from build123d import *

# Parameters (mm, degrees)
F0_W     = 42.2
F0_H     = 42
F1_DEPTH = 6
F3_R     = 1
F4_R     = 1
F5_DEPTH = 3
F6_R     = 1.65
F7_DEPTH = 6.001


with BuildPart() as f1:
    # F0 (on Top) → F1 (new body)
    with BuildSketch(Plane.XY):
        Rectangle(F0_W, F0_H)
        with BuildLine():
            Line((13, -8), (-13, -8))
            ThreePointArc((-13, -8), (-15.5, -5.5), (-13, -3))
            Line((-13, -3), (13, -3))
            ThreePointArc((13, -3), (15.5, -5.5), (13, -8))
        make_face(mode=Mode.SUBTRACT)
        with BuildLine():
            Line((13, 3), (-13, 3))
            ThreePointArc((-13, 3), (-15.5, 5.5), (-13, 8))
            Line((-13, 8), (13, 8))
            ThreePointArc((13, 8), (15.5, 5.5), (13, 3))
        make_face(mode=Mode.SUBTRACT)
    extrude(amount=F1_DEPTH)

    # F3
    f3_edges = [f1.edges().sort_by_distance(p)[0] for p in [
        (-21.1, -21, 3),
        (21.1, -21, 3),
        (-21.1, 21, 3),
        (21.1, 21, 3),
    ]]
    fillet(f3_edges, radius=F3_R)

    # F4
    f4_edges = [f1.edges().sort_by_distance(p)[0] for p in [
        (0, -21, 0),
        (0, -3, 0),
        (0, 8, 0),
    ]]
    fillet(f4_edges, radius=F4_R)

    # F2 (on face) → F5 (cut)
    with BuildSketch(Plane(origin=(0, 0, 0), x_dir=(1, 0, 0), z_dir=(0, 0, -1))):
        Polygon((-12.5, 13.767949), (-12.5, 17.232051), (-15.5, 18.964102), (-18.5, 17.232051), (-18.5, 13.767949), (-15.5, 12.035898), align=None)
        Polygon((12.5, 17.232051), (12.5, 13.767949), (15.5, 12.035898), (18.5, 13.767949), (18.5, 17.232051), (15.5, 18.964102), align=None)
        Polygon((12.5, -13.767949), (12.5, -17.232051), (15.5, -18.964102), (18.5, -17.232051), (18.5, -13.767949), (15.5, -12.035898), align=None)
        Polygon((-12.5, -17.232051), (-12.5, -13.767949), (-15.5, -12.035898), (-18.5, -13.767949), (-18.5, -17.232051), (-15.5, -18.964102), align=None)
    extrude(amount=-F5_DEPTH, mode=Mode.SUBTRACT)

    # F6 (on face) → F7 (cut, through all)
    with BuildSketch(Plane(origin=(0, 0, 0), x_dir=(1, 0, 0), z_dir=(0, 0, -1))):
        with Locations((-15.5, 15.5)):
            Circle(F6_R)
        with Locations((15.5, 15.5)):
            Circle(F6_R)
        with Locations((15.5, -15.5)):
            Circle(F6_R)
        with Locations((-15.5, -15.5)):
            Circle(F6_R)
    extrude(amount=-F7_DEPTH, mode=Mode.SUBTRACT)


solid = f1.part
The listing builds one solid part. Answer for the finished solid, in the listing's coordinates (mm). A direction names the side the tool comes from. Coordinates: 2 decimals unless noted, no trailing zeros. Loops run counter-clockwise (first coordinate to the right, second up) from the corner with the lowest first, then second, coordinate; pieces in that order, holes last. Notation, with made-up numbers: M -32.75,-32.5 L 23.25,-32.5 A29 ccw 23.25,-12.5 Z; hole C -10.75,3.25 d11. An arc over 180 degrees is marked long. Answer in a Markdown table with one row per item.
1) Find section B-B (y = -15.5). Determine the outline of the cut face in (x, z), then the cut area to 3 significant figures.
Answers below:
| item | result |
|---|---|
| outline | M -21.1,1 A1 ccw -20.1,0 L -18.5,0 L -18.5,3 L -17.15,3 L -17.15,6 L -21.1,6 Z; M -13.85,3 L -12.5,3 L -12.5,0 L 12.5,0 L 12.5,3 L 13.85,3 L 13.85,6 L -13.85,6 Z; M 17.15,3 L 18.5,3 L 18.5,0 L 20.1,0 A1 ccw 21.1,1 L 21.1,6 L 17.15,6 Z |
| area | 197 mm^2 |
2) Find section A-A (z = 4.75). Determine the outline of the cut face in (x, y), then the cut area to 3 significant figures.
Answers below:
| item | result |
|---|---|
| outline | M -21.1,-20 A1 ccw -20.1,-21 L 20.1,-21 A1 ccw 21.1,-20 L 21.1,20 A1 ccw 20.1,21 L -20.1,21 A1 ccw -21.1,20 Z; hole C -15.5,-15.5 d3.3; hole C -15.5,15.5 d3.3; hole M -13,-8 L 13,-8 A2.5 ccw 13,-3 L -13,-3 A2.5 ccw Z; hole M -13,3 L 13,3 A2.5 ccw 13,8 L -13,8 A2.5 ccw Z; hole C 15.5,-15.5 d3.3; hole C 15.5,15.5 d3.3 |
| area | 1,440 mm^2 |
3) Determine the mould class of faces 1 (the flat face through (-12.5, -15, 1)), 2 (the cylindrical face through (20.799, -20.715, 3.535)), 3 (the flat face through (0, 21, 3)) for opening direction X: released by +X, released by -X, zero draft, split by the parting line, or undercut.
Answers below:
| item | result |
|---|---|
| face 1 | undercut |
| face 2 | released by +X |
| face 3 | zero draft |
4) Find section C-C (y = -5.5). Determine the outline of the cut face in (x, z).
Answers below:
| item | result |
|---|---|
| outline | M -21.1,1 A1 ccw -20.1,0 L -16.5,0 A1 ccw -15.5,1 L -15.5,6 L -21.1,6 Z; M 15.5,1 A1 ccw 16.5,0 L 20.1,0 A1 ccw 21.1,1 L 21.1,6 L 15.5,6 Z |
5) Which of the six approach directions +Z, -Z, +X, -X, +Y, -Y give full straight-line access (tool end or side, diameter ignored) to faces 4 (the flat face through (0, -8, 3)), 5 (the cylindrical face through (20.799, 0.28, 0.285)), 6 (the flat face through (-14, 12.9, 1.5))?
Answers below:
| item | result |
|---|---|
| face 4 | +Z, -Z |
| face 5 | -Z, +X, +Y, -Y |
| face 6 | -Z |
6) Find section D-D (y = 15). Determine the outline of the cut face in (x, z), then the cut area to 3 significant figures.
Answers below:
| item | result |
|---|---|
| outline | M -21.1,1 A1 ccw -20.1,0 L -18.5,0 L -18.5,3 L -17.07,3 L -17.07,6 L -21.1,6 Z; M -13.93,3 L -12.5,3 L -12.5,0 L 12.5,0 L 12.5,3 L 13.93,3 L 13.93,6 L -13.93,6 Z; M 17.07,3 L 18.5,3 L 18.5,0 L 20.1,0 A1 ccw 21.1,1 L 21.1,6 L 17.07,6 Z |
| area | 198 mm^2 |
7) Find the intervals of material crossed by probe 1 along X at (y, z) = (-15.5, 4.8); probe 2 along Y at (x, z) = (-2.5, 2.55); probe 3 along X at (y, z) = (-16, 0.95), in increasing order.
Answers below:
| item | result |
|---|---|
| probe 1 | -21.1 to -17.15, -13.85 to 13.85, 17.15 to 21.1 |
| probe 2 | -21 to -8, -3 to 3, 8 to 21 |
| probe 3 | -21.1 to -18.5, -12.5 to 12.5, 18.5 to 21.1 |
8) Given pin 1 (5.5 mm diameter, centred on x = 15.5, y = -15.5, fed in from -Z); pin 2 (2 mm diameter, centred on x = 15.5, y = 15.5, fed in from +Z), each flat-ended and moving along its own axis, determine where each tip first touches the part or whether it passes through.
Answers below:
| item | result |
|---|---|
| pin 1 | z = 3 |
| pin 2 | through |
